Can you work these out from the model? Positions are in its coordinate system, mm. A direction names the side the tool comes from. Coordinates: 2 decimals unless noted, no trailing zeros. Order: outer loops, then holes, each group sorted by start corner. A loop starts at its lowest first (then second) coordinate and runs counter-clockwise, first axis right, second up. Notation, with made-up numbers: (-29, 18.5) -> (-21, 18.5) arc R18 cw to (-21, 40.5) -> close; hole circle Ø5 at (-30, 76.5). An arc over 180 degrees is marked (long way). Answer in a Markdown table with one row per item.
Autodesk Inventor part; units mm, degrees
ref_plane "YZ Plane" through (0, 0, 0) normal (1, 0, 0) x (0, 1, 0)
ref_plane "XZ Plane" through (0, 0, 0) normal (0, 1, 0) x (-1, 0, 0)
ref_plane "XY Plane" through (0, 0, 0) normal (0, 0, 1) x (1, 0, 0)
sketch "Skizze1" plane through (0, 0, 0) normal (0, 1, 0) x (-1, 0, 0)
  line L0 (-5.15, 2.75) -> (2.65, 2.75)
  line L1 (2.65, 2.75) -> (2.65, 0)
  line L2 (2.65, 0) -> (5.15, 0)
  line L3 (5.15, 0) -> (5.15, -2.75)
  line L4 (5.15, -2.75) -> (-5.15, -2.75)
  line L5 (-5.15, -2.75) -> (-5.15, 2.75)
  line L6 (8.4, 6) -> (-8.4, 6)
  line L7 (-8.4, 6) -> (-8.4, -6)
  line L8 (-8.4, -6) -> (8.4, -6)
  line L9 (8.4, -6) -> (8.4, 6)
  line L10 (8.4, 6) -> (-8.4, -6) construction
  line L11 (-8.4, 6) -> (8.4, -6) construction
  point P0 (0, 0)
  point P1 (0, 0)
  dimension "d0" = 16.8
  dimension "d1" = 12
  dimension "d2" = 5.5
  dimension "d3" = 10.3
  dimension "d4" = 2.75
  dimension "d5" = 7.8
  dimension "d6" = 2.75
  dimension "d7" = 3.25
  dimension "d8" = 3.25
extrude "Extrusion1" add sketch "Skizze1" along normal blind 6
fillet "Rundung1" radius 4 4 edges at (8.4, 3, -6) (8.4, 3, 6) (-8.4, 3, -6) (-8.4, 3, 6)
sketch "Skizze3" plane through (4.4, 0, -6) normal (0, 0, -1) x (-1, 0, 0)
  line L0 (8.075, 3) -> (6.525, 3)
  line L1 (6.525, 3) -> (4.3724, -0.2522)
  line L2 (8.075, 3) -> (5.9224, -0.2522)
  line L3 (8.075, 3) -> (11.975, 3) construction
  line L4 (5.9224, -0.2522) -> (4.3724, -0.2522)
  line L5 (3.0224, -0.2522) -> (7.3276, 6.2522)
  line L6 (3.0224, -0.2522) -> (10.8224, -0.2522) construction
  line L7 (7.3276, 6.2522) -> (5.7776, 6.2522)
  line L8 (7.3276, 6.2522) -> (8.8776, 6.2522) construction
  line L9 (5.7776, 6.2522) -> (1.4724, -0.2522)
  line L10 (1.4724, -0.2522) -> (3.0224, -0.2522)
  line L11 (4.4276, 6.2522) -> (2.8776, 6.2522)
  line L12 (2.8776, 6.2522) -> (0.725, 3)
  line L13 (0.725, 3) -> (2.275, 3)
  line L14 (0.725, 3) -> (2.275, 3) construction
  line L15 (2.275, 3) -> (4.4276, 6.2522)
  line L16 (-4, 6) -> (-4, 0)
  line L17 (12.8, 0) -> (12.8, 6)
  line L18 (0, 6) -> (8.8, 6)
  line L19 (0, 0) -> (8.8, 0)
  point P0 (4.4, 0)
  point P1 (0, 9.9522)
  dimension "d21" = 3.9
  dimension "d22" = 123.5
  dimension "d23" = 3.9
  dimension "d24" = 123.5
  dimension "d25" = 7.8
  dimension "d26" = 56.5
  dimension "d27" = 1.55
  dimension "d28" = 1.55
  dimension "d29" = 1.55
  dimension "d30" = 180
  dimension "d31" = 123.5
  dimension "d32" = 1.55
  dimension "d33" = 3.9
  dimension "d34" = 123.5
  dimension "d35" = 1.55
  dimension "d36" = 0
  dimension "d37" = 1.35
  dimension "d38" = 1.35
  dimension "d39" = 7.35
  dimension "d42" = 3.7
  dimension "d43" = 0
  dimension "d50" = 4.725
  dimension "d51" = 4.725
  dimension "d52" = -0.2521
  dimension "d53" = 0.2521
extrude "Extrusion3" cut sketch "Skizze3" against normal blind 0.5
chamfer "Fase2" distance 0.5 angle 45 2 edges at (-2.9, 3, -5.5) (2.9, 3, -5.5)
equation "\"d0\" = d3 + 2 * d7"
equation "\"d7\" = d8"
equation "\"d37\" = d38"
equation "\"d50\" = d51"
properties part number "Piholder"
(1) We'd pull the mould along X, two halves only. Please class faces 4 (the flat face through (8.4, 3, 0)), 5 (the flat face through (-0.75, 2.96, -5.75)), 6 (the flat face through (1.6, 3, -6)): +X half, -X half, draft (parallel to the pull), parting line (faces both ways), or undercut.
Response values:
| item | result |
|---|---|
| face 4 | +X half |
| face 5 | undercut |
| face 6 | draft |
(2) Suppose I cut it at C-C (x = 6.25). Please give me the cut outline in (y, z), and give its area (3 significant figures).
Response values:
| item | result |
|---|---|
| outline | (0, -5.55) -> (6, -5.55) -> (6, 5.55) -> (0, 5.55) -> close |
| area | 66.6 mm2 |
(3) On a 3-axis mill with a long thin cutter (end or side, diameter ignored), from which of +Z, -Z, +X, -X, +Y, -Y can I reach the whole of each face in a straight line? I mean faces 1 (the flat face through (-5.15, 3, -1)), 2 (the flat face through (-2.696, 1.521, -5.754)), 3 (the cylindrical face through (7.197, 3.042, 4.859)). Say none if no direction works.
Response values:
| item | result |
|---|---|
| face 1 | +Y, -Y |
| face 2 | -Z |
| face 3 | +Z, +X, +Y, -Y |
(4) Suppose I cut it at B-B (y = 2.05). Please give me the cut outline in (x, z).
Response values:
| item | result |
|---|---|
| outline | (-8.4, -2) arc R4 ccw to (-4.4, -6) -> (-3.05, -6) -> (-3.05, -5.5) -> (-1.5, -5.5) -> (-1.5, -6) -> (-0.15, -6) -> (-0.15, -5.5) -> (1.4, -5.5) -> (1.4, -6) -> (4.4, -6) arc R4 ccw to (8.4, -2) -> (8.4, 2) arc R4 ccw to (4.4, 6) -> (-4.4, 6) arc R4 ccw to (-8.4, 2) -> close; hole (-5.15, -2.75) -> (5.15, -2.75) -> (5.15, 2.75) -> (-2.65, 2.75) -> (-2.65, 0) -> (-5.15, 0) -> close |
(5) Suppose I cut it at D-D (z = 5.5). Please give me the cut outline in (x, y), and give its area (3 significant figures).
Response values:
| item | result |
|---|---|
| outline | (-6.34, 0) -> (6.34, 0) -> (6.34, 6) -> (-6.34, 6) -> close |
| area | 76.0 mm2 |
(6) I need wall thicknesses on line 1 (X direction, y = 2.8, z = -1.5); line 2 (Z direction, x = 2.75, y = 2.3); line 3 (Z direction, x = 0.5, y = 2.45). Which ranges of each line are inside material? Lowest first, please. Write a range as [from, to].
Response values:
| item | result |
|---|---|
| line 1 | [-8.4, -5.15], [5.15, 8.4] |
| line 2 | [-6, -2.75], [2.75, 6] |
| line 3 | [-5.5, -2.75], [2.75, 6] |
(7) Suppose I cut it at A-A (z = -0.5). Please give me the cut outline in (x, y).
Response values:
| item | result |
|---|---|
| outline | (-8.4, 0) -> (-5.15, 0) -> (-5.15, 6) -> (-8.4, 6) -> close; (5.15, 0) -> (8.4, 0) -> (8.4, 6) -> (5.15, 6) -> close |
